Model file for the job. Use its own axes, mm. A direction names the side the tool comes from. Give positions to 0.01 mm unless a question says otherwise; leave off trailing zeros. Loops run counter-clockwise (first coordinate to the right, second up) from the corner with the lowest first, then second, coordinate; pieces in that order, holes last. Notation, with made-up numbers: (75.25, -10.5) - (80.25, -10.5) arc R25 ccw to (80.25, 11.5) - close; hole circle Ø4 at (47.25, 12.25). An arc over 180 degrees is marked (long way). Answer as CSV lines item,"result". Start each with the question number.
Item 1: Saw through at B-B on y = 0.25. Give the cut face in (x, z) (3 decimals), plus the area to 3 significant figures.
Item 2: Pull direction Y, two halves, no side cores. Call faces 3 (the flat face through (7.62, 0, 6)), 4 (the flat face through (0, -5.08, 6)), 5 (the flat face through (0, -4.445, 7)): pulls with the +Y half, pulls with the -Y half, needs draft (parallel to the pull), parting line crosses it, or undercut.
Item 3: Tool access for faces 1 (the flat face through (0, 0, 0)), 2 (the flat face through (6.985, 0, 7)): list every direction of +Z, -Z, +X, -X, +Y, -Y with a clear straight run to the whole face (end or side of a thin tool).
Item 4: Drill centre lines: L1, parallel to Y at x = 1, z = 3.5 (3 decimals); L2, parallel to X at y = 2.75, z = 12 (3 decimals); L3, parallel to Z at x = 6.25, y = 1.5. Where is each one in solid material? Low to high. Write a range as from..to.
Item 5: Saw through at A-A on z = 11.25. Give the cut face in (x, y) (3 decimals).
Item 6: Saw through at C-C on x = 4. Give the cut face in (y, z) (3 decimals).
Item 7: Pin check, flat tip, straight feed: pin 1 (3 mm diameter, centred on x = -3.5, y = -1, fed in from +Z). Stop position of the tip, or through.
from build123d import *

# Parameters (mm, degrees)
F0_W     = 15.24
F0_H     = 10.16
F1_DEPTH = 12.7
F2_W     = 13.97
F2_H     = 8.89
F3_DEPTH = 11.43
F4_W     = 2.54
F4_H     = 0.5442967311
F5_DEPTH = 2.54


with BuildPart() as f1:
    # F0 (on Top) → F1 (new body)
    with BuildSketch(Plane.XY):
        Rectangle(F0_W, F0_H)
    extrude(amount=F1_DEPTH)

    # F2 (on face) → F3 (cut)
    with BuildSketch(Plane.XY.offset(12.7)):
        Rectangle(F2_W, F2_H)
    extrude(amount=-F3_DEPTH, mode=Mode.SUBTRACT)

    # F4 (on face) → F5 (cut)
    with BuildSketch(Plane.XZ.offset(5.08)):
        with Locations((0, 12.4278516345)):
            Rectangle(F4_W, F4_H)
    extrude(amount=-F5_DEPTH, mode=Mode.SUBTRACT)


solid = f1.part
Responses:
1,outline,"(-7.62, 0) - (7.62, 0) - (7.62, 12.7) - (6.985, 12.7) - (6.985, 1.27) - (-6.985, 1.27) - (-6.985, 12.7) - (-7.62, 12.7) - close"
1,area,"33.9 mm2"
2,face 3,"needs draft"
2,face 4,"pulls with the -Y half"
2,face 5,"undercut"
3,face 1,"-Z, +X, -X, +Y, -Y"
3,face 2,"+Z"
4,L1,"-5.08..-4.445, 4.445..5.08"
4,L2,"-7.62..-6.985, 6.985..7.62"
4,L3,"0..1.27"
5,outline,"(-7.62, -5.08) - (7.62, -5.08) - (7.62, 5.08) - (-7.62, 5.08) - close; hole (-6.985, -4.445) - (6.985, -4.445) - (6.985, 4.445) - (-6.985, 4.445) - close"
6,outline,"(-5.08, 0) - (5.08, 0) - (5.08, 12.7) - (4.445, 12.7) - (4.445, 1.27) - (-4.445, 1.27) - (-4.445, 12.7) - (-5.08, 12.7) - close"
7,pin 1,"z = 1.27"
